Can you work these out from the model? Positions are in its coordinate system, mm. A direction names the side the tool comes from. Round coordinates to 2 decimals unless told otherwise and drop trailing zeros. Loops run counter-clockwise (first coordinate to the right, second up) from the corner with the lowest first, then second, coordinate; pieces in that order, holes last. Notation, with made-up numbers: (-7.75, -18) -> (29.25, -18) arc R19 cw to (29.25, 16) -> close; hole circle Ø8 at (-22, 54.5). An arc over 180 degrees is marked (long way). Write item = value, one per line.
from build123d import *

# Parameters (mm, degrees)
F0_W           = 431.8
F0_H           = 50.8
F1_DEPTH       = 20.7264
F2_W           = 25.4
F2_H           = 9.525
F3_DEPTH       = 25.4
F4_W           = 25.4
F4_H           = 9.525
F5_DEPTH       = 25.4
F6_R           = 6.35
F8_D           = 6.35
F8_CBORE_D     = 12.7
F8_CBORE_DEPTH = 3.175


with BuildPart() as f1:
    # F0 (on Front) → F1 (new body)
    with BuildSketch(Plane.XZ):
        with Locations((20.574, -37.44022)):
            Rectangle(F0_W, F0_H)
    extrude(amount=F1_DEPTH)

    # F2 (on face) → F3 (join)
    with BuildSketch(Plane(origin=(0, 0, -62.84022), x_dir=(1, 0, 0), z_dir=(0, 0, -1))):
        with Locations((-182.626, 4.7625)):
            Rectangle(F2_W, F2_H)
        with Locations((223.774, 4.7625)):
            Rectangle(F2_W, F2_H)
    extrude(amount=F3_DEPTH)

    # F4 (on face) → F5 (join)
    with BuildSketch(Plane.XY.offset(-12.04022)):
        with Locations((-182.626, -4.7625)):
            Rectangle(F4_W, F4_H)
        with Locations((223.774, -4.7625)):
            Rectangle(F4_W, F4_H)
    extrude(amount=F5_DEPTH)

    # F6
    f6_edges = [f1.edges().sort_by_distance(p)[0] for p in [
        (236.474, -4.7625, -88.24022),
        (211.074, -4.7625, -88.24022),
        (236.474, -4.7625, 13.35978),
        (211.074, -4.7625, 13.35978),
        (-169.926, -4.7625, 13.35978),
        (-195.326, -4.7625, 13.35978),
        (-195.326, -4.7625, -88.24022),
        (-169.926, -4.7625, -88.24022),
    ]]
    fillet(f6_edges, radius=F6_R)

    # F8 (through all)
    with Locations(Plane.XZ.offset(9.525)):
        with Locations((-182.626, 0.65978), (-182.626, -75.54022), (223.774, 0.65978), (223.774, -75.54022)):
            CounterBoreHole(F8_D / 2, F8_CBORE_D / 2, F8_CBORE_DEPTH)


solid = f1.part
1. I'm going to push flat-ended pins straight in: pin 1 (10 mm diameter, centred on x = 223.77, z = 0.66, fed in from -Y); pin 2 (10 mm diameter, centred on x = 226.5, z = 3, fed in from -Y) (3 decimals); pin 3 (5.5 mm diameter, centred on x = 223.77, z = -75.54, fed in from -Y); pin 4 (5 mm diameter, centred on x = -120, y = -8.5, fed in from -Z). Where does each tip first touch, or does it pass through?
Entries:
pin_1 = -6.35
pin_2 = -9.525
pin_3 = through
pin_4 = -62.84
2. Suppose I cut it at A-A, the plane x = 174.5. List the corners of the cut face in (y, z) for me.
Entries:
outline = (-20.73, -62.84) -> (0, -62.84) -> (0, -12.04) -> (-20.73, -12.04) -> close
3. Suppose I cut it at B-B, the plane y = -14.5. List the corners of the cut face in (x, z) for me.
Entries:
outline = (-195.33, -62.84) -> (236.47, -62.84) -> (236.47, -12.04) -> (-195.33, -12.04) -> close
4. For faces 4 (the flat face through (220.8, -9.525, -69.7)), 5 (the flat face through (-169.926, -5, -3)), 6 (the flat face through (211.074, -5, -72)), 7 (the flat face through (224, -5, 13.36)), 8 (the flat face through (225, -6.35, 4)), which set-ups out of +Z, -Z, +X, -X, +Y, -Y let a thin tool reach every point of the face, with its end or its side?
Entries:
face_4 = -Z, +X, -X, -Y
face_5 = +Z, +Y, -Y
face_6 = -Z, +Y, -Y
face_7 = +Z, +X, -X, +Y, -Y
face_8 = -Y
5. We'd pull the mould along Z, two halves only. Please class faces 1 (the flat face through (-183, -5, 13.36)), 2 (the flat face through (-183, -5, -88.24)), 3 (the cylindrical face through (217.43, -7.96, -75.26)): released by +Z, released by -Z, zero draft, split by the parting line, or undercut.
Entries:
face_1 = released by +Z
face_2 = released by -Z
face_3 = undercut
6. I need wall thicknesses on line 1 (X direction, y = -7.75, z = -2); line 2 (Z direction, x = -75.5, y = -5.5); line 3 (X direction, y = -2.5, z = -81.5). Which ranges of each line are inside material? Lowest first, please. Write a range as [from, to].
Entries:
line_1 = [-195.33, -188.39], [-176.86, -169.93], [211.07, 218.01], [229.54, 236.47]
line_2 = [-62.84, -12.04]
line_3 = [-195.33, -169.93], [211.07, 236.47]
